CAD build for the part. Positions are in the model's coordinates, mm. Round coordinates to 2 decimals unless told otherwise and drop trailing zeros. Loops run counter-clockwise (first coordinate to the right, second up) from the corner with the lowest first, then second, coordinate; pieces in that order, holes last. Notation, with made-up numbers: (14, -8) - (60, -8) arc R12 ccw to (60, 12) - close; hole circle Ø1 at (-26, -10). An arc over 180 degrees is marked (long way). One line per question, with ' | ' between items.
```python
from build123d import *

# Parameters (mm, degrees)
SKETCH1_R           = 5.55625
BOSS_EXTRUDE1_DEPTH = 1.651
SKETCH5_R           = 2.38125
CUT_EXTRUDE1_DEPTH  = 2.651
FILLET1_R           = 0.2032


with BuildPart() as part:
    # Sketch1 → Boss-Extrude1 (new body)
    with BuildSketch(Plane(origin=(0, 0, 0), x_dir=(1, 0, 0), z_dir=(0, 1, 0))):
        Circle(SKETCH1_R)
    extrude(amount=BOSS_EXTRUDE1_DEPTH)

    # Sketch5 → Cut-Extrude1 (cut, through all)
    with BuildSketch(Plane(origin=(0, 1.651, 0), x_dir=(-1, 0, 0), z_dir=(0, 1, 0))):
        Circle(SKETCH5_R)
    extrude(amount=-CUT_EXTRUDE1_DEPTH, mode=Mode.SUBTRACT)

    # Fillet1
    fillet1_edges = [part.edges().sort_by_distance(p)[0] for p in [
        (-5.55625, 0, 0),
        (-5.55625, 1.651, 0),
        (2.38125, 0, 0),
        (2.38125, 1.651, 0),
    ]]
    fillet(fillet1_edges, radius=FILLET1_R)


solid = part.part
```
(1) Probe L1, parallel to Z at x = 0, y = 1.15; L2, parallel to X at y = 0.95, z = 1.5; L3, parallel to Z at x = 2, y = 0.1. List the from-to ranges inside material, lowest first.
Results found:
L1: z = -5.56 to -2.38, 2.38 to 5.56 | L2: x = -5.35 to -1.85, 1.85 to 5.35 | L3: z = -5.15 to -1.34, 1.34 to 5.15
(2) Cut at C-C, the plane y = 1.2. Write the cut outline in (x, z).
Results found:
outline: circle Ø11.11 at (0, 0); hole circle Ø4.76 at (0, 0)
(3) Drop a flat-ended pin along its axis: P1, Ø4.5, axis at x = 0, z = 0, coming from the +Y side. Give the stop position or say it passes through.
Results found:
P1: passes through
(4) Cut at A-A, the plane z = 0. Write the cut outline in (x, y), then the cut area to 3 significant figures.
Results found:
outline: (-5.56, 0.2) arc R0.2 ccw to (-5.35, 0) - (-2.58, 0) arc R0.2 ccw to (-2.38, 0.2) - (-2.38, 1.45) arc R0.2 ccw to (-2.58, 1.65) - (-5.35, 1.65) arc R0.2 ccw to (-5.56, 1.45) - close; (2.38, 0.2) arc R0.2 ccw to (2.58, 0) - (5.35, 0) arc R0.2 ccw to (5.56, 0.2) - (5.56, 1.45) arc R0.2 ccw to (5.35, 1.65) - (2.58, 1.65) arc R0.2 ccw to (2.38, 1.45) - close | area: 10.4 mm²
(5) Cut at B-B, the plane x = 0. Write the cut outline in (y, z).
Results found:
outline: (0, -5.35) arc R0.2 ccw to (0.2, -5.56) - (1.45, -5.56) arc R0.2 ccw to (1.65, -5.35) - (1.65, -2.58) arc R0.2 ccw to (1.45, -2.38) - (0.2, -2.38) arc R0.2 ccw to (0, -2.58) - close; (0, 2.58) arc R0.2 ccw to (0.2, 2.38) - (1.45, 2.38) arc R0.2 ccw to (1.65, 2.58) - (1.65, 5.35) arc R0.2 ccw to (1.45, 5.56) - (0.2, 5.56) arc R0.2 ccw to (0, 5.35) - close
(6) Two-plate mould, pull along X, no slides. Class faces 1 (the face through (1.89, 0.83, -1.45)), 2 (the face through (5.3, 0.82, -1.67)), 3 (the face through (-1.3, 0, -2.5)): released by +X, released by -X, zero draft, split by the parting line, or undercut.
Results found:
face 1: undercut | face 2: split by the parting line | face 3: zero draft
